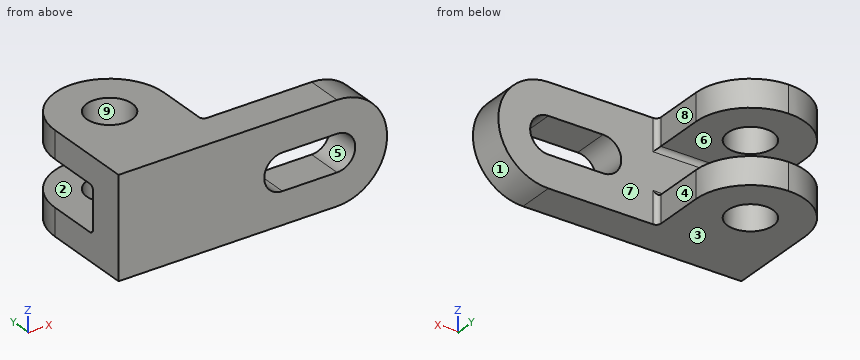
```python
from build123d import *

# Parameters (mm, degrees)
BOSS_EXTRUDE1_DEPTH = 40.64
SKETCH2_W           = 121.92
SKETCH2_H           = 30.48
BOSS_EXTRUDE3_DEPTH = 121.92
CUT_EXTRUDE1_DEPTH  = 40.64
CUT_EXTRUDE3_DEPTH  = 111.76
SKETCH5_5_R         = 25.4
CUT_EXTRUDE4_DEPTH  = 111.76
FILLET1_R           = 5.08


with BuildPart() as part:
    # Sketch1 → Boss-Extrude1 (new body)
    with BuildSketch(Plane(origin=(0, 0, 0), x_dir=(1, 0, 0), z_dir=(0, 1, 0))):
        with BuildLine():
            Line((-43.798165138, 94.906788991), (200.041834862, 94.906788991))
            ThreePointArc((200.041834862, 94.906788991), (255.921834862, 39.026788991), (200.041834862, -16.853211009))
            Line((200.041834862, -16.853211009), (-43.798165138, -16.853211009))
            Line((-43.798165138, -16.853211009), (-43.798165138, 94.906788991))
        make_face()
    extrude(amount=BOSS_EXTRUDE1_DEPTH)

    # Sketch2 → Boss-Extrude3 (add)
    with BuildSketch(Plane(origin=(0, 40.64, 0), x_dir=(1, 0, 0), z_dir=(0, 1, 0))):
        with Locations((17.161834862, -1.613211009)):
            Rectangle(SKETCH2_W, SKETCH2_H)
        with Locations((17.161834862, 79.666788991)):
            Rectangle(SKETCH2_W, SKETCH2_H)
    extrude(amount=BOSS_EXTRUDE3_DEPTH)

    # Sketch2<6> → Cut-Extrude1 (cut)
    with BuildSketch(Plane(origin=(0, 40.64, 0), x_dir=(1, 0, 0), z_dir=(0, 1, 0))):
        with BuildLine():
            Line((200.041834862, 59.346788991), (139.081834862, 59.346788991))
            ThreePointArc((139.081834862, 59.346788991), (118.761834862, 39.026788991), (139.081834862, 18.706788991))
            Line((139.081834862, 18.706788991), (200.041834862, 18.706788991))
            ThreePointArc((200.041834862, 18.706788991), (220.361834862, 39.026788991), (200.041834862, 59.346788991))
        make_face()
    extrude(amount=-CUT_EXTRUDE1_DEPTH, mode=Mode.SUBTRACT)

    # Sketch5 → Cut-Extrude3 (cut)
    with BuildSketch(Plane.XY.offset(16.853211009)):
        with BuildLine():
            Line((78.121834862, 162.56), (17.161834862, 162.56))
            ThreePointArc((17.161834862, 162.56), (60.267064244, 144.705229381), (78.121834862, 101.6))
            Line((78.121834862, 101.6), (78.121834862, 162.56))
        make_face()
        with BuildLine():
            Line((-43.798165138, 162.56), (-43.798165138, 101.6))
            ThreePointArc((-43.798165138, 101.6), (-25.943394519, 144.705229381), (17.161834862, 162.56))
            Line((17.161834862, 162.56), (-43.798165138, 162.56))
        make_face()
    extrude(amount=-CUT_EXTRUDE3_DEPTH, mode=Mode.SUBTRACT)

    # Sketch5<5> → Cut-Extrude4 (cut)
    with BuildSketch(Plane.XY.offset(16.853211009)):
        with Locations((17.161834862, 101.6)):
            Circle(SKETCH5_5_R)
    extrude(amount=-CUT_EXTRUDE4_DEPTH, mode=Mode.SUBTRACT)

    # Fillet1
    fillet1_edges = [part.edges().sort_by_distance(p)[0] for p in [
        (17.161834862, 40.64, -13.626788991),
        (78.121834862, 40.64, 1.613211009),
        (78.121834862, 40.64, -79.666788991),
        (17.161834862, 40.64, -64.426788991),
    ]]
    fillet(fillet1_edges, radius=FILLET1_R)


solid = part.part
```
Model file for the job. Use its own axes, mm. Face numbers are marked on the shaded views. A direction names the side the tool comes from. Coordinates: 2 decimals unless noted, no trailing zeros. Loops run counter-clockwise (first coordinate to the right, second up) from the corner with the lowest first, then second, coordinate; pieces in that order, holes last. Notation, with made-up numbers: (6, 82) -> (61, 82) arc R18 ccw to (61, 112) -> close; hole circle Ø11 at (71.5, 31.25). An arc over 180 degrees is marked (long way). Answer as a JSON object with one key per item and string values.
Q1. Flat gauge pins, fed straight in: P1, Ø5, axis at y = 38.5, z = -60, coming from the +X side; P2, Ø15, axis at y = 65.5, z = -72, coming from the +X side; P3, Ø8, axis at x = 69.5, z = -83.5, coming from the +Y side. Where does each tip first touch, or does it go through?
Report:
{"P1": "stops at x = 252.78", "P2": "stops at x = 78.12", "P3": "stops at y = 138.74"}
Q2. Probe probe 1 along X at (y, z) = (101, -74); probe 2 along Z at (x, y) = (-22, 78); probe 3 along Z at (x, y) = (149, 24.5). List the from-to ranges inside material, lowest first.
Report:
{"probe 1": "x = -43.8 to -8.23, 42.55 to 78.12", "probe 2": "z = -94.91 to -64.43, -13.63 to 16.85", "probe 3": "z = -94.91 to -59.35, -18.71 to 16.85"}
Q3. Cut at B-B (x = 195.5). List the corners of the cut face in (y, z).
Report:
{"outline": "(0, -94.91) -> (40.64, -94.91) -> (40.64, -59.35) -> (0, -59.35) -> close; (0, -18.71) -> (40.64, -18.71) -> (40.64, 16.85) -> (0, 16.85) -> close"}
Q4. 3-axis set-ups, long thin cutter, end or side, ignore diameter. For the marked faces 5, 6, 7, 8 and 9: which of +Z, -Z, +X, -X, +Y, -Y reach the whole face in a straight line?
Report:
{"face 5": "+Y, -Y", "face 6": "+X, -X, +Y", "face 7": "+X, +Y", "face 8": "+Z, -Z, +X, +Y", "face 9": "+Z, -Z"}
Q5. Cut at C-C (z = -25). List the corners of the cut face in (x, y), and give its area (3 significant figures).
Report:
{"outline": "(-43.8, 0) -> (124.38, 0) -> (124.38, 40.64) -> (-43.8, 40.64) -> close; (214.74, 0) -> (254.13, 0) -> (254.13, 40.64) -> (214.74, 40.64) -> close", "area": "8,440 mm2"}
Q6. Pull direction Z, two halves, no side cores. Call the marked faces 1, 2, 3 and 4: released by +Z, released by -Z, zero draft, split by the parting line, or undercut.
Report:
{"face 1": "split by the parting line", "face 2": "undercut", "face 3": "released by -Z", "face 4": "zero draft"}
Q7. Cut at D-D (z = -83). List the corners of the cut face in (x, y).
Report:
{"outline": "(-43.8, 0) -> (234.52, 0) -> (234.52, 40.64) -> (83.2, 40.64) arc R5.08 cw to (78.12, 45.72) -> (78.12, 101.6) arc R60.96 ccw to (-43.8, 101.6) -> close; hole circle Ø50.8 at (17.16, 101.6)"}
Q8. Cut at A-A (y = 35). List the corners of the cut face in (x, z).
Report:
{"outline": "(-43.8, -94.91) -> (200.04, -94.91) arc R55.88 ccw to (200.04, 16.85) -> (-43.8, 16.85) -> close; hole (139.08, -59.35) -> (200.04, -59.35) arc R20.32 ccw to (200.04, -18.71) -> (139.08, -18.71) arc R20.32 ccw to start"}
